Source: CAD feature listing. Evaluate the final solid. Frame: model axes, mm. A direction names the side the tool comes from. Round coordinates to 2 decimals unless told otherwise and drop trailing zeros. Loops run counter-clockwise (first coordinate to the right, second up) from the corner with the lowest first, then second, coordinate; pieces in that order, holes last. Notation, with made-up numbers: M 48.5,-4 L 91.5,-4 A26 ccw 91.5,12 Z; hole C -7.5,37.5 d11. An arc over 180 degrees is marked long. Answer as a JSON object with one key per item and string values.
from build123d import *

# Parameters (mm, degrees)
SKETCH037_W     = 47
SKETCH037_H     = 42.3
PAD022_DEPTH    = 42.3
SKETCH038_R     = 1.5
POCKET020_DEPTH = 4.5
SKETCH039_R     = 11
PAD023_DEPTH    = 2
SKETCH040_R     = 2.5
PAD024_DEPTH    = 24


with BuildPart() as part:
    # Sketch037 → Pad022 (new body)
    with BuildSketch(Plane.XY):
        Rectangle(SKETCH037_W, SKETCH037_H)
    extrude(amount=PAD022_DEPTH)

    # Sketch038 (on Face4 of Pad022) → Pocket020 (cut)
    with BuildSketch(Plane(origin=(-23.5, 0, 0), x_dir=(0, -1, 0), z_dir=(-1, 0, 0))):
        with Locations((-15.5, 36.65)):
            Circle(SKETCH038_R)
        with Locations((15.5, 36.65)):
            Circle(SKETCH038_R)
        with Locations((-15.5, 5.65)):
            Circle(SKETCH038_R)
        with Locations((15.5, 5.65)):
            Circle(SKETCH038_R)
    extrude(amount=-POCKET020_DEPTH, mode=Mode.SUBTRACT)

    # Sketch039 (on Face2 of Pocket020) → Pad023 (join)
    with BuildSketch(Plane(origin=(-23.5, 0, 0), x_dir=(0, -1, 0), z_dir=(-1, 0, 0))):
        with Locations((0, 21.15)):
            Circle(SKETCH039_R)
    extrude(amount=PAD023_DEPTH)

    # Sketch040 (on Face13 of Pad023) → Pad024 (join)
    with BuildSketch(Plane(origin=(-25.5, 0, 0), x_dir=(0, -1, 0), z_dir=(-1, 0, 0))):
        with Locations((0, 21.15)):
            Circle(SKETCH040_R)
    extrude(amount=PAD024_DEPTH)


solid = part.part
Item 1: Section C-C on x = -40. Return the cut outline in (y, z), then the cut area to 3 significant figures.
Answer sheet:
{"outline": "C 0,21.15 d5", "area": "19.6 mm²"}
Item 2: Line query: probe 1 along Z at (x, y) = (-21.5, 15.5); probe 2 along Y at (x, z) = (-22, 5); probe 3 along X at (y, z) = (13, 18.5). Output: solid intervals per line, ascending. Write a range as from..to.
Answer sheet:
{"probe 1": "z = 0..4.15, 7.15..35.15, 38.15..42.3", "probe 2": "y = -21.15..-16.85, -14.15..14.15, 16.85..21.15", "probe 3": "x = -23.5..23.5"}
Item 3: Access query for faces 5 (the flat face through (0, 21.15, 21)), 6 (the flat face through (-23.5, -10, 11)). Directions: +Z, -Z, +X, -X, +Y, -Y. A direction counts if a zero-diameter tool reaches every point of the face in a straight line with its end or side. Return the directions, or none.
Answer sheet:
{"face 5": "+Z, -Z, +X, -X, +Y", "face 6": "-X"}
Item 4: Section D-D on y = -7. Return the cut outline in (x, z).
Answer sheet:
{"outline": "M -25.5,12.66 L -23.5,12.66 L -23.5,0 L 23.5,0 L 23.5,42.3 L -23.5,42.3 L -23.5,29.64 L -25.5,29.64 Z"}
Item 5: Contact query for flat-ended pins moving along their axis: pin 1 Ø12.5 at (y, z) = (5, 29) entering from -X; pin 2 Ø4 at (y, z) = (-15.5, 36.65) entering from -X; pin 3 Ø0.9 at (y, z) = (-15.5, 5.5) entering from -X. Output: stop coordinate, or through.
Answer sheet:
{"pin 1": "stops at x = -25.5", "pin 2": "stops at x = -23.5", "pin 3": "stops at x = -19"}
Item 6: Section B-B on z = 21.15. Return the cut outline in (x, y).
Answer sheet:
{"outline": "M -49.5,-2.5 L -25.5,-2.5 L -25.5,-11 L -23.5,-11 L -23.5,-21.15 L 23.5,-21.15 L 23.5,21.15 L -23.5,21.15 L -23.5,11 L -25.5,11 L -25.5,2.5 L -49.5,2.5 Z"}
Item 7: Pull-direction query (Z, two-part tool) for faces 1 (the flat face through (-19, -15, 6)), 2 (the flat face through (0, -21.15, 21)), 3 (the cylindrical face through (-37.33, 0.33, 23.63)), 4 (the flat face through (-19, 16, 6)); classes: pulls with the +Z half, pulls with the -Z half, needs draft (parallel to the pull), parting line crosses it, or undercut.
Answer sheet:
{"face 1": "undercut", "face 2": "needs draft", "face 3": "parting line crosses it", "face 4": "undercut"}
Item 8: Section A-A on y = 0. Return the cut outline in (x, z), then the cut area to 3 significant figures.
Answer sheet:
{"outline": "M -49.5,18.65 L -25.5,18.65 L -25.5,10.15 L -23.5,10.15 L -23.5,0 L 23.5,0 L 23.5,42.3 L -23.5,42.3 L -23.5,32.15 L -25.5,32.15 L -25.5,23.65 L -49.5,23.65 Z", "area": "2,150 mm²"}
